from build123d import *

# Parameters (mm, degrees)
SKETCH2_W                 = 80
SKETCH2_H                 = 211
BOSS_EXTRUDE1_DEPTH       = 2
M3X0_5_TAPPED_HOLE1_D     = 2.5
M3X0_5_TAPPED_HOLE1_DEPTH = 10
M3X0_5_TAPPED_HOLE1_TIP   = 0.751075774
SKETCH7_R                 = 3
CUT_EXTRUDE1_DEPTH        = 2


with BuildPart() as part:
    # Sketch2 → Boss-Extrude1 (new body)
    with BuildSketch(Plane.XY):
        with Locations((40, 105.5)):
            Rectangle(SKETCH2_W, SKETCH2_H)
    extrude(amount=BOSS_EXTRUDE1_DEPTH)

    # M3x0.5 Tapped Hole1
    with Locations(Plane(origin=(0, 0, 0), x_dir=(-1, 0, 0), z_dir=(0, 0, -1))):
        with Locations((-75, 196), (-5, 196), (-75, 23), (-5, 23)):
            Hole(M3X0_5_TAPPED_HOLE1_D / 2, depth=M3X0_5_TAPPED_HOLE1_DEPTH)
            with Locations((0, 0, -(M3X0_5_TAPPED_HOLE1_DEPTH + M3X0_5_TAPPED_HOLE1_TIP / 2))):  # 118° drill point
                Cone(0, M3X0_5_TAPPED_HOLE1_D / 2, M3X0_5_TAPPED_HOLE1_TIP, mode=Mode.SUBTRACT)

    # Sketch7 → Cut-Extrude1 (cut)
    with BuildSketch(Plane(origin=(0, 0, 0), x_dir=(-1, 0, 0), z_dir=(0, 0, -1))):
        with Locations((-75, 186)):
            Circle(SKETCH7_R)
        with Locations((-75, 139.2)):
            Circle(SKETCH7_R)
        with Locations((-75, 109.2)):
            Circle(SKETCH7_R)
        with Locations((-75, 79.2)):
            Circle(SKETCH7_R)
        with Locations((-75, 59.2)):
            Circle(SKETCH7_R)
        with Locations((-75, 33.2)):
            Circle(SKETCH7_R)
        with Locations((-5, 186)):
            Circle(SKETCH7_R)
        with Locations((-5, 139.2)):
            Circle(SKETCH7_R)
        with Locations((-5, 109.2)):
            Circle(SKETCH7_R)
        with Locations((-5, 79.2)):
            Circle(SKETCH7_R)
        with Locations((-5, 59.2)):
            Circle(SKETCH7_R)
        with Locations((-5, 33.2)):
            Circle(SKETCH7_R)
        with Locations((-70.3, 13)):
            Circle(SKETCH7_R)
        with Locations((-60, 205)):
            Circle(SKETCH7_R)
        with Locations((-20, 205)):
            Circle(SKETCH7_R)
        with Locations((-60, 6)):
            Circle(SKETCH7_R)
        with Locations((-20, 6)):
            Circle(SKETCH7_R)
        with Locations((-9.7, 13)):
            Circle(SKETCH7_R)
    extrude(amount=-CUT_EXTRUDE1_DEPTH, mode=Mode.SUBTRACT)


solid = part.part
Can you work these out from the model? Positions are in its coordinate system, mm. Give positions to 0.01 mm unless a question says otherwise; leave off trailing zeros. Loops run counter-clockwise (first coordinate to the right, second up) from the corner with the lowest first, then second, coordinate; pieces in that order, holes last. Notation, with made-up numbers: (6, -22) -> (11, -22) arc R26 ccw to (11, 0) -> close; hole circle Ø10 at (-6.75, -22.75). An arc over 180 degrees is marked (long way). Write item = value, one per line.
1) Suppose I cut it at A-A on y = 139.2. Write out the boundary of the cut face in (x, z), then the cut area to 3 significant figures.
Check result:
outline = (0, 0) -> (2, 0) -> (2, 2) -> (0, 2) -> close; (8, 0) -> (72, 0) -> (72, 2) -> (8, 2) -> close; (78, 0) -> (80, 0) -> (80, 2) -> (78, 2) -> close
area = 136 mm2
2) I need wall thicknesses on L1, parallel to X at y = 186, z = 1.2; L2, parallel to X at y = 196, z = 1.35; L3, parallel to Y at x = 60, z = 0.8. Which ranges of each line are inside material? Lowest first, please. Write a range as from..to.
Check result:
L1 = 0..2, 8..72, 78..80
L2 = 0..3.75, 6.25..73.75, 76.25..80
L3 = 0..3, 9..202, 208..211
3) Will this pin go through, and if not, where does the flat tip stop? pin 1 (5.5 mm diameter, centred on x = 60, y = 6, fed in from -Z).
Check result:
pin_1 = through
4) Suppose I cut it at C-C on z = 1.5. Give the number of separate pieces and of enclosed holes in the cut face, then the cut area to 3 significant figures.
Check result:
separate_pieces = 1
enclosed_holes = 22
area = 16,400 mm2
5) Suppose I cut it at B-B on x = 60. Write out the boundary of the cut face in (y, z), then the cut area to 3 significant figures.
Check result:
outline = (0, 0) -> (3, 0) -> (3, 2) -> (0, 2) -> close; (9, 0) -> (202, 0) -> (202, 2) -> (9, 2) -> close; (208, 0) -> (211, 0) -> (211, 2) -> (208, 2) -> close
area = 398 mm2
6) Thinking about a two-plate mould opening in X: for faces 1 (the cylindrical face through (77.4, 137.4, 1)), 2 (the flat face through (39, 107, 0)), 3 (the cylindrical face through (5.391, 112.174, 0.986)), which applies, released by +X, released by -X, zero draft, split by the parting line, or undercut?
Check result:
face_1 = undercut
face_2 = zero draft
face_3 = undercut
